Input: part model. Units: mm. Frame: model coordinates. A direction names the side the tool comes from. Give positions to 0.01 mm unless a question says otherwise; leave off trailing zeros. Loops run counter-clockwise (first coordinate to the right, second up) from the corner with the lowest first, then second, coordinate; pieces in that order, holes last. Notation, with made-up numbers: M -26.5,19 L -11.5,19 A19 ccw -11.5,37 Z; hole C 69,64 d3. An arc over 180 degrees is marked long. Use a Markdown table: item, result. Add a question column.
from build123d import *

# Parameters (mm, degrees)
EXTRUDE_1_DEPTH     = 5
FILLET_2_R          = 2
SKETCH_2_R          = 7
EXTRUDE_2_DEPTH     = 5
SKETCH_2_2_R        = 7
CUT_EXTRUDE_1_DEPTH = 2
SKETCH_3_R          = 3.5
CUT_EXTRUDE_2_DEPTH = 53.297030326
SKETCH_4_R          = 13
EXTRUDE_3_DEPTH     = 13
SKETCH_5_R          = 9
CUT_EXTRUDE_3_DEPTH = 54.8050126
SKETCH_6_R          = 2.5
CUT_EXTRUDE_4_DEPTH = 53.820255404
CHAMFER_1_SIZE      = 0.5
FILLET_1_R          = 2


with BuildPart() as part:
    # Sketch 1 → Extrude 1 (new body)
    with BuildSketch(Plane(origin=(0, 0, 0), x_dir=(1, 0, 0), z_dir=(0, 1, 0))):
        with BuildLine():
            Line((-16.363068172, 27.5), (16.363068172, 27.5))
            ThreePointArc((16.363068172, 27.5), (0, -32), (-16.363068172, 27.5))
        make_face()
    extrude(amount=EXTRUDE_1_DEPTH)

    # Fillet 2
    fillet_2_edges = [part.edges().sort_by_distance(p)[0] for p in [
        (0, 5, 32),
        (0, 5, -27.5),
    ]]
    fillet(fillet_2_edges, radius=FILLET_2_R)

    # Sketch 2 → Extrude 2 (add)
    with BuildSketch(Plane(origin=(0, 5, 0), x_dir=(1, 0, 0), z_dir=(0, 1, 0))):
        with Locations((0, -32)):
            Circle(SKETCH_2_R)
        with Locations((-27.712812921, 16)):
            Circle(SKETCH_2_R)
        with Locations((27.712812921, 16)):
            Circle(SKETCH_2_R)
    extrude(amount=-EXTRUDE_2_DEPTH)

    # Sketch 2_2 → Cut-Extrude 1 (cut)
    with BuildSketch(Plane(origin=(0, 5, 0), x_dir=(1, 0, 0), z_dir=(0, 1, 0))):
        with Locations((0, -32)):
            Circle(SKETCH_2_2_R)
        with Locations((-27.712812921, 16)):
            Circle(SKETCH_2_2_R)
        with Locations((27.712812921, 16)):
            Circle(SKETCH_2_2_R)
    extrude(amount=-CUT_EXTRUDE_1_DEPTH, mode=Mode.SUBTRACT)

    # Sketch 3 → Cut-Extrude 2 (cut, through all)
    with BuildSketch(Plane(origin=(0, 3, 0), x_dir=(1, 0, 0), z_dir=(0, 1, 0))):
        with Locations(Location((0, -32, 0), (0, 0, 270))):
            Circle(SKETCH_3_R)
        with Locations(Location((-27.712812921, 16, 0), (0, 0, 270))):
            Circle(SKETCH_3_R)
        with Locations(Location((27.712812921, 16, 0), (0, 0, 270))):
            Circle(SKETCH_3_R)
    extrude(amount=-CUT_EXTRUDE_2_DEPTH, mode=Mode.SUBTRACT)

    # Sketch 4 → Extrude 3 (add)
    with BuildSketch(Plane(origin=(0, 0, 0), x_dir=(1, 0, 0), z_dir=(0, 1, 0))):
        with Locations(Location((0, 3.5, 0), (0, 0, 90))):
            Circle(SKETCH_4_R)
    extrude(amount=EXTRUDE_3_DEPTH)

    # Sketch 5 → Cut-Extrude 3 (cut, through all)
    with BuildSketch(Plane(origin=(0, 13, 0), x_dir=(1, 0, 0), z_dir=(0, 1, 0))):
        with Locations(Location((0, 3.5, 0), (0, 0, 270))):
            Circle(SKETCH_5_R)
    extrude(amount=-CUT_EXTRUDE_3_DEPTH, mode=Mode.SUBTRACT)

    # Sketch 6 → Cut-Extrude 4 (cut, through all)
    with BuildSketch(Plane(origin=(0, 5, 0), x_dir=(1, 0, 0), z_dir=(0, 1, 0))):
        with Locations(Location((27.5, 6, 0), (0, 0, 270))):
            Circle(SKETCH_6_R)
        with Locations(Location((-27.5, 6, 0), (0, 0, 211.537077351))):
            Circle(SKETCH_6_R)
    extrude(amount=-CUT_EXTRUDE_4_DEPTH, mode=Mode.SUBTRACT)

    # Chamfer 1
    chamfer_1_edges = [part.edges().sort_by_distance(p)[0] for p in [
        (0, 13, -12.5),
    ]]
    chamfer(chamfer_1_edges, length=CHAMFER_1_SIZE)

    # Fillet 1
    fillet_1_edges = [part.edges().sort_by_distance(p)[0] for p in [
        (0, 5, 9.5),
        (0, 13, 9.5),
    ]]
    fillet(fillet_1_edges, radius=FILLET_1_R)


solid = part.part
1) Pull-direction query (X, two-part tool) for faces 1 (the flat face through (0, 0, 6)), 2 (the cylindrical face through (-33.69, 1.52, -19.64)), 3 (the cylindrical face through (27.896, 1.479, 15.678)); classes: pulls with the +X half, pulls with the -X half, needs draft (parallel to the pull), parting line crosses it, or undercut.
2) Section query D-D, the plane z = -6. State how many separate pieces and enclosed holes the cut face has, and give its area (3 significant figures).
3) Reachability of faces 4 (the flat face through (0, 5, 14)), 5 (the flat face through (3, 3, 35)), 6 (the cylindrical face through (-20.231, 1.479, -24.793)), 7 (the cylindrical face through (-25, 3, -6)) from +Z, -Z, +X, -X, +Y, -Y: full face, straight path, thin tool, end or side. Return the list, or none.
4) Section query C-C, the plane y = 8. Return the cut outline in (x, z), and give its area (3 significant figures).
5) Contact query for flat-ended pins moving along their axis: P1, Ø1, axis at y = 3.5, z = -6.5, coming from the +X side; P2, Ø11, axis at x = 3, z = 35.5, coming from the +Y side; P3, Ø14.5, axis at x = 0, z = -3.5, coming from the +Y side; P4, Ø11, axis at x = -25.5, z = -13, coming from the +Y side. Output: stop coordinate, or through.
6) Section query B-B, the plane y = 1.75. Return the cut outline in (x, z), and give its area (3 significant figures).
7) Section query A-A, the plane x = 0. Return the cut outline in (y, z).
8) Ray query, line 1 (Z direction, x = 27.5, y = 2.4); line 2 (X direction, y = 1, z = -5.5); line 3 (X direction, y = 3.75, z = -6). Return the intervals inside material, ascending. Write a range as [from, to].
Entries:
| question | item | result |
|---|---|---|
| 1 | face 1 | needs draft |
| 1 | face 2 | undercut |
| 1 | face 3 | pulls with the +X half |
| 2 | separate pieces | 4 |
| 2 | enclosed holes | 0 |
| 2 | area | 242 mm² |
| 3 | face 4 | +Y |
| 3 | face 5 | +Z, +Y |
| 3 | face 6 | -Z, +Y, -Y |
| 3 | face 7 | +Y, -Y |
| 4 | outline | C 0,-3.5 d26; hole C 0,-3.5 d18 |
| 4 | area | 276 mm² |
| 5 | P1 | stops at x = 31.4 |
| 5 | P2 | stops at y = 3 |
| 5 | P3 | passes through |
| 5 | P4 | stops at y = 5 |
| 6 | outline | M -30.53,-9.59 A7 ccw long -23.57,-21.64 A32 ccw -16.36,-27.5 L 16.36,-27.5 A32 ccw 23.57,-21.64 A7 ccw long 30.53,-9.59 A32 ccw 6.96,31.23 A7 ccw long -6.96,31.23 A32 ccw Z; hole C -27.71,-16 d7; hole C -27.5,-6 d5; hole C 0,-3.5 d18; hole C 0,32 d7; hole C 27.71,-16 d7; hole C 27.5,-6 d5 |
| 6 | area | 2,950 mm² |
| 7 | outline | M 0,-27.5 L 3,-27.5 A2 ccw 5,-25.5 L 5,-18.5 A2 cw 7,-16.5 L 11,-16.5 A2 ccw 13,-14.5 L 13,-13 L 12.5,-12.5 L 0,-12.5 Z; M 0,5.5 L 12.5,5.5 L 13,6 L 13,7.5 A2 ccw 11,9.5 L 7,9.5 A2 cw 5,11.5 L 5,25 L 3,25 L 3,28.5 L 0,28.5 Z; M 0,35.5 L 3,35.5 L 3,39 L 0,39 Z |
| 8 | line 1 | z = [-23, -19.49], [-12.51, -8.5], [-3.5, 16.36] |
| 8 | line 2 | x = [-31.52, -29.95], [-25.05, -8.77], [8.77, 25.05], [29.95, 31.52] |
| 8 | line 3 | x = [-31.28, -30], [-25, -8.65], [8.65, 25], [30, 31.28] |
